```python
from build123d import *

# Parameters (mm, degrees)
F1_DEPTH      = 2.5
F2_R          = 3.5
F3_DEPTH      = 75
F5_DEPTH      = 2
F7_DEPTH      = 40
F7_DEPTH_BACK = 15
F8_R          = 0.8


with BuildPart() as f1:
    # F0 (on Top) → F1 (new body)
    with BuildSketch(Plane.XY):
        with BuildLine():
            ThreePointArc((0, -2), (-0.585786, -0.585786), (-2, 0))
            Line((-2, 0), (-108, 0))
            ThreePointArc((-108, 0), (-109.414214, -0.585786), (-110, -2))
            Line((-110, -2), (-110, -158))
            ThreePointArc((-110, -158), (-109.414214, -159.414214), (-108, -160))
            Line((-108, -160), (-52, -160))
            ThreePointArc((-52, -160), (-50.585786, -159.414214), (-50, -158))
            Line((-50, -158), (-50, -90))
            ThreePointArc((-50, -90), (-38.284271, -61.715729), (-10, -50))
            Line((-10, -50), (-2, -50))
            ThreePointArc((-2, -50), (-0.585786, -49.414214), (0, -48))
            Line((0, -48), (0, -2))
        make_face()
    extrude(amount=F1_DEPTH)

    # F2 (on face) → F3 (join)
    with BuildSketch(Plane(origin=(0, 0, 0), x_dir=(1, 0, 0), z_dir=(0, 0, -1))):
        with Locations((-78.837842, 141.606882)):
            Circle(F2_R)
        with Locations((-78.837842, 23.552824)):
            Circle(F2_R)
    extrude(amount=F3_DEPTH)

    # F4 (on face) → F5 (join)
    with BuildSketch(Plane(origin=(0, 0, -75), x_dir=(1, 0, 0), z_dir=(0, 0, -1))):
        with BuildLine():
            ThreePointArc((-56.533181, 137.606882), (-52.533181, 141.606882), (-56.533181, 145.606882))
            Line((-56.533181, 145.606882), (-104.533181, 145.606882))
            ThreePointArc((-104.533181, 145.606882), (-108.533181, 141.606882), (-104.533181, 137.606882))
            Line((-104.533181, 137.606882), (-56.533181, 137.606882))
        make_face()
        with BuildLine():
            ThreePointArc((-82.337842, 141.606882), (-78.837842, 145.106882), (-75.337842, 141.606882))
            ThreePointArc((-75.337842, 141.606882), (-78.837842, 138.106882), (-82.337842, 141.606882))
        make_face(mode=Mode.SUBTRACT)
        with BuildLine():
            ThreePointArc((-104.533181, 27.552824), (-108.533181, 23.552824), (-104.533181, 19.552824))
            Line((-104.533181, 19.552824), (-15.066023, 19.552824))
            ThreePointArc((-15.066023, 19.552824), (-11.066023, 23.552824), (-15.066023, 27.552824))
            Line((-15.066023, 27.552824), (-104.533181, 27.552824))
        make_face()
        with BuildLine():
            ThreePointArc((-82.337842, 23.552824), (-78.837842, 27.052824), (-75.337842, 23.552824))
            ThreePointArc((-75.337842, 23.552824), (-78.837842, 20.052824), (-82.337842, 23.552824))
        make_face(mode=Mode.SUBTRACT)
        with BuildLine():
            ThreePointArc((-82.337842, 23.552824), (-78.837842, 20.052824), (-75.337842, 23.552824))
            Line((-75.337842, 23.552824), (-82.337842, 23.552824))
        make_face()
    extrude(amount=-F5_DEPTH)

    # F6 (on face) → F7 (join, two sides)
    with BuildSketch(Plane.XY.offset(2.5)) as f7_sk:
        Polygon((-108, 0), (-88, 0), (-88, 1), (-111, 1), (-111, -82), (-110, -82), (-110, -2), (-110, 0), align=None)
    extrude(amount=F7_DEPTH)
    extrude(f7_sk.sketch, amount=-F7_DEPTH_BACK)

    # F8
    f8_edges = [f1.edges().sort_by_distance(p)[0] for p in [
        (-111, 1, 15),
    ]]
    fillet(f8_edges, radius=F8_R)


solid = f1.part
```
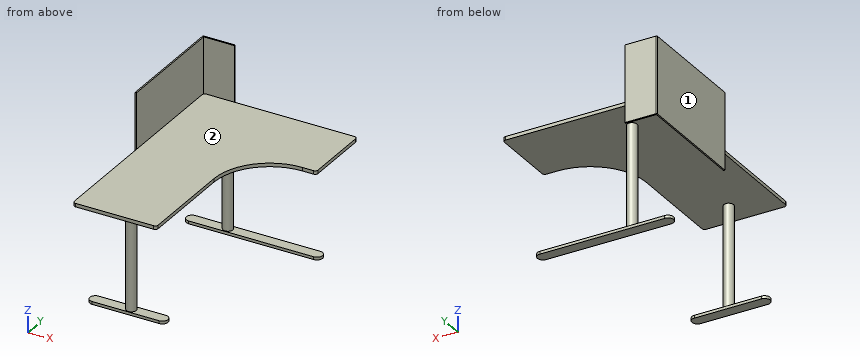
Verification items for the finished model (mm, model axes). Face numbers are marked on the shaded views. A direction names the side the tool comes from. Coordinates: 2 decimals unless noted, no trailing zeros. Order: outer loops, then holes, each group sorted by start corner. A loop starts at its lowest first (then second) coordinate and runs counter-clockwise, first axis right, second up. Notation, with made-up numbers: (81.5, -21) -> (110.5, -21) arc R33 cw to (110.5, 9) -> close; hole circle Ø9 at (77.5, -5.5). An arc over 180 degrees is marked (long way). Put each result on its own line as item: value. Start each with the question number.
1) Cross-section at B-B (y = -46). Enter the section's corners in (x, z).
2) Tool access check on the marked faces 1 and 2. Record the directions out of +Z, -Z, +X, -X, +Y, -Y that give a thin tool (end or side, any length) a straight path to the whole face; none if there is none.
3) Cross-section at D-D (x = -22.5). Enter the section's corners in (y, z).
4) Cross-section at C-C (z = 29.5). Enter the section's corners in (x, y), plus the area to 3 significant figures.
5) Go/stop test with flat-tipped pins: pin 1 (2 mm diameter, centred on x = -76, z = -74.5, fed in from -Y); pin 2 (8 mm diameter, centred on x = -50, y = -111.5, fed in from -Z); pin 3 (8 mm diameter, centred on y = -23.5, z = 11, fed in from +X). Record where each tip stops, or that it passes through.
6) Material ranges on L1, parallel to Z at x = -69, y = -143; L2, parallel to X at y = -148, z = 2; L3, parallel to Z at x = -26, y = -38.5, recorded low to high.
7) Cross-section at A-A (x = -59.5). Enter the section's corners in (y, z).
Geometry check:
1. outline: (-111, -12.5) -> (-110, -12.5) -> (-110, 0) -> (0, 0) -> (0, 2.5) -> (-110, 2.5) -> (-110, 42.5) -> (-111, 42.5) -> close
2. face 1: +Z, -Z, -X, +Y, -Y
2. face 2: +Z, +X, -Y
3. outline: (-52, 0) -> (0, 0) -> (0, 2.5) -> (-52, 2.5) -> close; (-27.55, -75) -> (-19.55, -75) -> (-19.55, -73) -> (-27.55, -73) -> close
4. outline: (-111, -82) -> (-110, -82) -> (-110, 0) -> (-88, 0) -> (-88, 1) -> (-110.2, 1) arc R0.8 ccw to (-111, 0.2) -> close
4. area: 105 mm^2
5. pin 1: stops at y = -145.61
5. pin 2: stops at z = 0
5. pin 3: stops at x = -110
6. L1: z = -75 to -73, 0 to 2.5
6. L2: x = -110 to -50
6. L3: z = 0 to 2.5
7. outline: (-160, 0) -> (0, 0) -> (0, 2.5) -> (-160, 2.5) -> close; (-145.61, -75) -> (-137.61, -75) -> (-137.61, -73) -> (-145.61, -73) -> close; (-27.55, -75) -> (-19.55, -75) -> (-19.55, -73) -> (-27.55, -73) -> close
